Part print with two shaded views. Sizes in mm from the minimum x, y, z corner. A direction names the side the tool comes from. Give positions to 0.01 mm unless a question says otherwise; leave off trailing zeros. Order: outer loops, then holes, each group sorted by start corner. A loop starts at its lowest first (then second) coordinate and runs counter-clockwise, first axis right, second up. Notation, with made-up numbers: (55, 75) -> (84, 75) arc R19 ccw to (84, 104) -> close; hole circle Ø3 at (5, -17). An arc over 180 degrees is marked (long way). Write item = value, one per line. Start each with the question number.
Item 1: Tool access for the marked faces 1 and 2: list every direction of +Z, -Z, +X, -X, +Y, -Y with a clear straight run to the whole face (end or side of a thin tool).
Item 2: Drill centre lines: line 1 along Z through (x, y) = (1.45, 4.5); line 2 along Y through (x, z) = (0.35, 6); line 3 along Y through (x, z) = (0.35, 7.5). Where is each one in solid material? Low to high.
Item 3: Band-saw the part on D-D on y = 11.75. Write the cut outline in (x, z), plus the area to 3 significant figures.
Item 4: Band-saw the part on A-A on y = 7. Write the cut outline in (x, z).
Item 5: Flat gauge pins, fed straight in: P1, Ø6, axis at y = 6, z = 11.5, coming from the -X side; P2, Ø1.5, axis at x = 2.5, y = 9.5, coming from the +Z side. Where does each tip first touch, or does it go through?
Item 6: Band-saw the part on C-C on x = 1.1. Write the cut outline in (y, z), plus the area to 3 significant figures.
Item 7: Pull direction Y, two halves, no side cores. Call the marked faces 3, 4, 5 and 6: +Y half, -Y half, draft (parallel to the pull), parting line (faces both ways), or undercut.
Item 8: Band-saw the part on B-B on z = 7. Write the cut outline in (x, y).
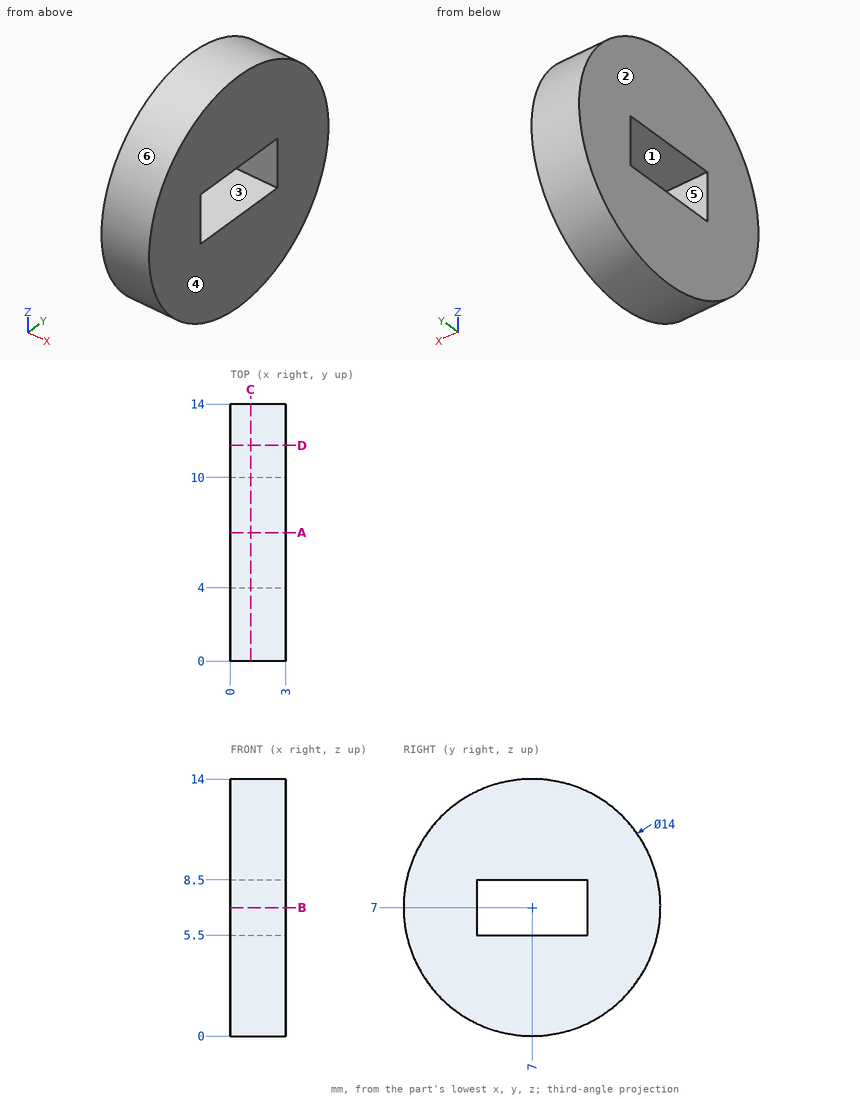
Values found:
q1.face_1 = +X, -X
q1.face_2 = +Z, -Z, -X, +Y, -Y
q2.line_1 = 0.46 to 5.5, 8.5 to 13.54
q2.line_2 = 0.07 to 4, 10 to 13.93
q2.line_3 = 0.02 to 4, 10 to 13.98
q3.outline = (0, 1.86) -> (3, 1.86) -> (3, 12.14) -> (0, 12.14) -> close
q3.area = 30.9 mm^2
q4.outline = (0, 0) -> (3, 0) -> (3, 5.5) -> (0, 5.5) -> close; (0, 8.5) -> (3, 8.5) -> (3, 14) -> (0, 14) -> close
q5.P1 = 0
q5.P2 = 13.78
q6.outline = circle Ø14 at (7, 7); hole (4, 5.5) -> (10, 5.5) -> (10, 8.5) -> (4, 8.5) -> close
q6.area = 136 mm^2
q7.face_3 = undercut
q7.face_4 = draft
q7.face_5 = undercut
q7.face_6 = parting line
q8.outline = (0, 0) -> (3, 0) -> (3, 4) -> (0, 4) -> close; (0, 10) -> (3, 10) -> (3, 14) -> (0, 14) -> close
